Autodesk Inventor part; units mm, degrees
ref_plane "Work Plane1" through (-1.0566, 20, -15.5001) normal (0, 1, 0) x (-0.6956, 0, 0.7184)
ref_plane "YZ Plane" through (0, 0, 0) normal (1, 0, 0) x (0, 1, 0)
ref_plane "XZ Plane" through (0, 0, 0) normal (0, 1, 0) x (-1, 0, 0)
sketch "Sketch1" plane through (0, 0, 0) normal (0, 1, 0) x (-1, 0, 0)
  arc A0 (-20.3357, 0) -> (-5.4696, 0) centre (-12.9027, 1) ccw
  circle A1 centre (-12.9027, 1) radius 7.5
  circle A2 centre (-12.9027, 1) radius 9.5
  line L0 (-0.4696, 0) -> (-5.4696, 0)
  line L1 (-20.3357, 0) -> (-25.3357, 0)
  line L2 (-0.4696, 0) -> (-25.3357, 0)
  line L3 (-25.3357, 0) -> (-25.3357, 1)
  line L4 (-25.3357, 1) -> (-0.4696, 1)
  line L5 (-0.4696, 1) -> (-0.4696, 0)
  line L6 (-0.4696, 1) -> (-25.3357, 1)
  line L7 (-25.3357, 1) -> (-25.3357, 3)
  line L8 (-25.3357, 3) -> (-0.4696, 3)
  line L9 (-0.4696, 3) -> (-0.4696, 1)
  line L10 (-25.3357, 3) -> (-16.9494, 9.9957)
  line L11 (-0.4696, 3) -> (-9.4027, 10.4518)
  point P0 (0, 0)
  point P1 (-6.8173, 8.2951)
  point P2 (-18.9881, 8.2951)
  point P3 (-20.4027, 1)
  point P4 (-5.4027, 1)
  dimension "d0" = 2
  dimension "d1" = 1
  dimension "d2" = 2
ref_plane "Work Plane1" through (-1.0566, 20, -15.5001) normal (0, 1, 0) x (-0.6956, 0, 0.7184)
extrude "Extrusion1" add sketch "Sketch1" along normal blind 20 and the other way blind 3 contours L4 A2 L8 A1 | A1 L8 A2 L4 | L8 A2 A1 | L4 L7 L8 A2 | A2 L8 L9 L4 | L8 L10 A2 | A2 L11 L8
ref_plane "Work Plane2" through (5.4027, -3, 3) normal (0, 0, -1) x (-1, 0, 0)
sketch "Sketch2" plane through (5.4027, -3, 3) normal (0, 0, -1) x (-1, 0, 0)
  circle A0 centre (2.433, 5) radius 1.15
  circle A1 centre (2.433, 18) radius 1.15
  line L0 (-0.067, 23) -> (-0.067, 0)
  line L1 (4.933, 23) -> (-0.067, 23)
  line L2 (4.933, 23) -> (4.933, 0)
  line L3 (-0.067, 0) -> (4.933, 0)
  circle A2 centre (-17.433, 18) radius 1.15
  circle A3 centre (-17.433, 5) radius 1.15
  line L4 (-14.933, 0) -> (-14.933, 23)
  line L5 (-19.933, 0) -> (-14.933, 0)
  line L6 (-19.933, 23) -> (-19.933, 0)
  line L7 (-14.933, 23) -> (-19.933, 23)
  circle A4 centre (2.433, 18) radius 2.3
  circle A5 centre (2.433, 5) radius 2.3
  circle A6 centre (-17.433, 18) radius 2.3
  circle A7 centre (-17.433, 5) radius 2.3
  point P0 (5.4027, 3)
  dimension "d6" = 4.6
  dimension "d7" = 4.6
  dimension "d8" = 4.6
  dimension "d9" = 4.6
extrude "Extrusion2" cut sketch "Sketch2" against normal blind 10 contours A0 | A1 | A2 | A3 | A4 | A5 | A6 | A7
hole "Hole1" at (2.9696, 15, 3) at (2.9696, 2, 3) at (22.8357, 2, 3) at (22.8357, 15, 3) direction (0, 0, -1) diameter 2.7 end through all
properties part number "cpap hose holder"
Check sheet for the modelled part. Datum: model origin and axes. Units: mm. A direction names the side the tool comes from. Round coordinates to 2 decimals unless told otherwise and drop trailing zeros. Loops run counter-clockwise (first coordinate to the right, second up) from the corner with the lowest first, then second, coordinate; pieces in that order, holes last. Notation, with made-up numbers: (38.5, 86.5) - (42.5, 86.5) arc R14 cw to (42.5, 98.5) - close; hole circle Ø1 at (-30, 28.25). An arc over 180 degrees is marked (long way). Answer as CSV lines item,"result". Start each with the question number.
Item 1: Section check B-B (y = 2). Record the boundary of the cut face in (x, z).
Item 2: Set-up check for faces 1 (the cylindrical face through (24.154, 2.293, 1.986)), 2 (the flat face through (21, 2, 3)): record each of +Z, -Z, +X, -X, +Y, -Y from which the full face is reachable in a straight line by a thin tool's end or side.
Item 3: Section check A-A (z = 2.25). Record the boundary of the cut face in (x, y), and give its area (3 significant figures).
Item 4: Section check D-D (x = 9.75). Record the boundary of the cut face in (y, z).
Item 5: Depth check by flat-ended pin: P1, Ø5, axis at x = 22.5, y = 3, coming from the +Z side; P2, Ø5, axis at x = 14.5, y = 11, coming from the -Z side; P3, Ø5, axis at x = 23.5, y = 14, coming from the +Z side (3 decimals); P4, Ø2.5, axis at x = 2.97, y = 15, coming from the +Z side. Enter the tip coordinate at first touch or a pass-through.
Item 6: Scan lines: line 1 (X direction, y = 2, z = 2.35); line 2 (X direction, y = 1.25, z = 2); line 3 (X direction, y = 15, z = 4). Record each from-to range of solid material in increasing order. Write a range as [from, to].
Item 7: Section check C-C (z = 6.5). Record the boundary of the cut face in (x, y).
Report:
1,outline,"(0.47, 1) - (1.62, 1) - (1.62, 3) - (0.67, 3) - (0.67, 3.17) - (0.47, 3) - close; (4.32, 1) - (5.4, 1) arc R7.5 cw to (20.4, 1) - (21.49, 1) - (21.49, 3) - (20.54, 3) - (20.54, 7) - (18.99, 8.3) arc R9.5 ccw to (6.82, 8.3) - (5.27, 7) - (5.27, 3) - (4.32, 3) - close; (24.19, 1) - (25.34, 1) - (25.34, 3) - (25.14, 3.17) - (25.14, 3) - (24.19, 3) - close"
2,face 1,"+Z, -Z"
2,face 2,"+Z"
3,outline,"(0.47, -3) - (5.51, -3) - (5.51, 20) - (0.47, 20) - close; (20.3, -3) - (25.34, -3) - (25.34, 20) - (20.3, 20) - close; hole circle Ø2.7 at (2.97, 2); hole circle Ø2.7 at (2.97, 15); hole circle Ø2.7 at (22.84, 2); hole circle Ø2.7 at (22.84, 15)"
3,area,"209 mm2"
4,outline,"(-3, 7.81) - (20, 7.81) - (20, 9.96) - (-3, 9.96) - close"
5,P1,"stops at z = 7.45"
5,P2,"stops at z = 7.28"
5,P3,"stops at z = 6.585"
5,P4,"passes through"
6,line 1,"x = [0.47, 1.62], [4.32, 5.53], [20.28, 21.49], [24.19, 25.34]"
6,line 2,"x = [0.47, 1.85], [4.09, 5.47], [20.34, 21.71], [23.96, 25.34]"
6,line 3,"x = [5.27, 6.03], [19.78, 20.54]"
7,outline,"(4.67, -3) - (7.8, -3) - (7.8, 20) - (4.67, 20) - (4.67, 16.55) arc R2.3 cw to (4.67, 13.45) - (4.67, 3.55) arc R2.3 cw to (4.67, 0.45) - close; (18, -3) - (21.14, -3) - (21.14, 0.45) arc R2.3 cw to (21.14, 3.55) - (21.14, 13.45) arc R2.3 cw to (21.14, 16.55) - (21.14, 20) - (18, 20) - close"
